Autodesk Inventor part; units mm, degrees
ref_plane "YZ Plane" through (0, 0, 0) normal (1, 0, 0) x (0, 1, 0)
ref_plane "XZ Plane" through (0, 0, 0) normal (0, 1, 0) x (-1, 0, 0)
ref_plane "XY Plane" through (0, 0, 0) normal (0, 0, 1) x (1, 0, 0)
sketch "Sketch1" plane through (0, 0, 0) normal (0, 0, 1) x (1, 0, 0)
  line L0 (0, 0) -> (34, 0)
  line L1 (34, 0) -> (34, 3)
  line L2 (34, 3) -> (0, 3)
  line L3 (0, 3) -> (0, 0)
  line L4 (0, 0) -> (-5.5, 0)
  line L5 (-5.5, 0) -> (-5.5, 1.5)
  line L6 (-5.5, 1.5) -> (0, 1.5)
  line L7 (0, 1.5) -> (0, 0)
  line L8 (34, 0) -> (44.5, 0)
  line L9 (44.5, 0) -> (44.5, 1.5)
  line L10 (44.5, 1.5) -> (34, 1.5)
  line L11 (34, 1.5) -> (34, 0)
  dimension "d0" = 3
  dimension "d1" = 34
  dimension "d2" = 1.5
  dimension "d3" = 5.5
  dimension "d4" = 1.5
  dimension "d5" = 10.5
revolve "Revolution1" add sketch "Sketch1" angle 360 about axis through (0, 0, 0) along (1, 0, 0)
fillet "Fillet1" radius 0.5 2 edges at (34, -1.5, 0) (0, -1.5, 0)
chamfer "Chamfer1" distance 0.5 angle 45 4 edges at (-5.5, -1.5, 0) (0, -3, 0) (34, -3, 0) (44.5, -1.5, 0)
sketch "Sketch2" plane through (0, 0, 0) normal (0, 1, 0) x (-1, 0, 0)
  line L0 (-14.7, 3) -> (-15.5, 3)
  line L1 (-15.5, 3) -> (-15.5, 2.85)
  line L2 (-15.5, 2.85) -> (-14.7, 2.85)
  line L3 (-14.7, 2.85) -> (-14.7, 3)
  line L4 (-0.5, -3) -> (-0.5, 3)
  line L5 (-33.5, 3) -> (-33.5, -3)
  line L6 (15.5, 0) -> (-54.5, 0)
  line L7 (0, 2.5) -> (0, -2.5)
  point P0 (0, 0)
  dimension "d11" = 2.85
  dimension "d12" = 0.8
  dimension "d13" = 15.5
revolve "Revolution2" cut sketch "Sketch2" angle 360 about axis through (-10, 0, 0) along (1, 0, 0)
equation "\"d4\" = d2"
properties part number "Pancake_Reverse Shaft" material "Aluminum 6061"
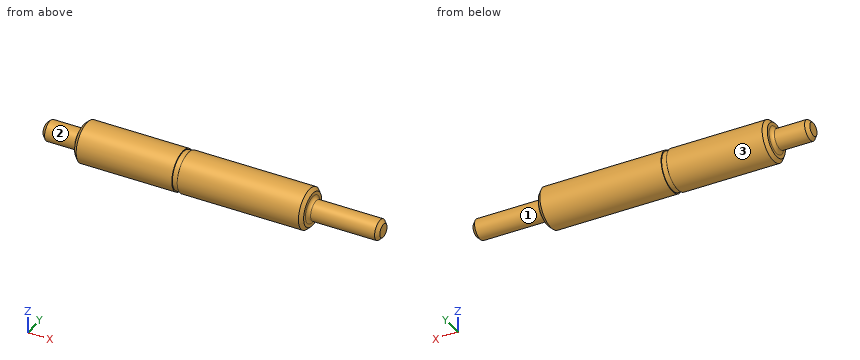
Read the model definition and answer for the solid it produces. Units are mm, in the model's axes. Face numbers are marked on the shaded views. A direction names the side the tool comes from. Give positions to 0.01 mm unless a question says otherwise; leave off trailing zeros. Write each loop counter-clockwise with the first axis right and the second up, starting at its lowest first coordinate (ties: lowest second). Pieces come first, ordered by that corner, then holes. Notation, with made-up numbers: (24.5, 79.25) - (75.5, 79.25) arc R33 ccw to (75.5, 107.25) - close; hole circle Ø1 at (-22, -24.75). An arc over 180 degrees is marked (long way). Return JSON: item names as keys, results as strings.
Q1. For the marked faces 1, 2 and 3, determine the directions among +Z, -Z, +X, -X, +Y, -Y from which every point of the face is accessible in a straight line to the end or side of a thin tool.
Reply:
{"face 1": "+X", "face 2": "-X", "face 3": "+X, -X"}
Q2. A cutting plane is placed at D-D, the plane x = 35.5. Determine the outline of the cut face in (y, z).
Reply:
{"outline": "circle Ø3 at (0, 0)"}
Q3. A cutting plane is placed at C-C, the plane x = 5.5. Determine the outline of the cut face in (y, z).
Reply:
{"outline": "circle Ø6 at (0, 0)"}
Q4. Consider line 1 along Y through (x, z) = (39, -0.1); line 2 along Z through (x, y) = (13, -1.25). Determine where each line is inside the solid, lowest interval first. Write a range as [from, to].
Reply:
{"line 1": "[-1.5, 1.5]", "line 2": "[-2.73, 2.73]"}
